Source: CAD feature listing. Evaluate the final solid. Frame: model axes, mm. A direction names the side the tool comes from. Round coordinates to 2 decimals unless told otherwise and drop trailing zeros. Write each loop counter-clockwise with the first axis right and the second up, starting at its lowest first coordinate (ties: lowest second). Pieces come first, ordered by that corner, then holes. Notation, with made-up numbers: M 86,37 L 129,37 A25 cw 129,72 Z; hole C -21,58.25 d10. An arc over 180 degrees is marked long. Use a Markdown table: item, result.
Autodesk Inventor part; units mm, degrees
ref_plane "YZ Plane" through (0, 0, 0) normal (1, 0, 0) x (0, 1, 0)
ref_plane "XZ Plane" through (0, 0, 0) normal (0, 1, 0) x (-1, 0, 0)
ref_plane "XY Plane" through (0, 0, 0) normal (0, 0, 1) x (1, 0, 0)
sketch "Sketch1" plane through (0, 0, 0) normal (0, 0, 1) x (1, 0, 0)
  line L0 (0, 0) -> (0, 12.75) construction
  line L1 (0, 0) -> (13.9342, 0) construction
  line L2 (0, 0) -> (0, -3)
  line L3 (0, -3) -> (12.5, -3)
  line L4 (12.5, -3) -> (12.5, 3.25)
  line L5 (12.5, 3.25) -> (9.075, 3.25)
  line L6 (9.075, 3.25) -> (9.075, 0)
  line L7 (9.075, 0) -> (0, 0)
  line L8 (3, 0) -> (5, 0)
  line L9 (5, 0) -> (5, -0.5)
  line L10 (5, -0.5) -> (3, -0.5)
  line L11 (3, -0.5) -> (3, 0)
  dimension "d0" = 3
  dimension "d1" = 5
  dimension "d2" = 0.5
  dimension "d3" = 9.075
  dimension "d4" = 12.5
  dimension "d5" = 3.25
  dimension "d6" = 3
revolve "Revolution1" add sketch "Sketch1" angle 360 about axis through (0, 0, 0) along (0, 1, 0) contours L7 L11 L10 L9 L6 L5 L4 L3 L2
chamfer "Chamfer1" distance 2 angle 45 1 edges at (-12.5, -3, 0)
chamfer "Chamfer2" distance 1 angle 45 1 edges at (-12.5, 3.25, 0)
sketch "Sketch2" plane through (0, 3.25, 0) normal (0, 1, 0) x (1, 0, 0)
  circle A0 centre (0, 0) radius 12.5
  circle A1 centre (0, 0) radius 12.5
  circle A2 centre (0, -12.5) radius 2.5
  line L0 (0, 0) -> (0, -12.5) construction
  point P0 (2.4875, -12.25)
  point P1 (-2.4875, -12.25)
  dimension "d14" = 5
extrude "Extrusion1" cut sketch "Sketch2" against normal through all contours A2 A0 picked at (0, -11.6481)
pattern_circular "Circular Pattern1" count 4 over 360 about axis through (0, -10, 0) along (0, 1, 0) of "Extrusion1"
sketch "Sketch3" plane through (0, 3.25, 12.5) normal (0, 1, 0) x (1, 0, 0)
  line L0 (0, 12.5) -> (0, -7.7808) construction
  line L1 (0, 12.5) -> (13.1543, -0.6543) construction
  circle A0 centre (7.4246, 5.0754) radius 0.75
  dimension "d20" = 45
  dimension "d21" = 1.5
  dimension "d22" = 10.5
extrude "Extrusion2" add sketch "Sketch3" along normal blind 1.5
chamfer "Chamfer3" distance 0.35 angle 45 1 edges at (6.6746, 4.75, 7.4246)
pattern_circular "Circular Pattern2" count 4 over 360 about axis through (0, -10, 0) along (0, 1, 0) of "Extrusion2", "Chamfer3"
properties part number "cpd_1.9_p0_v12"
Q1. Line query: L1, parallel to X at y = -0.15, z = 0; L2, parallel to Z at x = 0, y = 2.25 (3 decimals). Output: solid intervals per line, ascending.
Results are:
| item | result |
|---|---|
| L1 | -10 to -5, -3 to 3, 5 to 10 |
| L2 | -10 to -9.075, 9.075 to 10 |
Q2. Mould query, pull axis Z, two halves, no side actions, for faces 1 (the flat face through (0, -3, 0)), 2 (the conical face through (8.186, 3.076, -8.323)), 3 (the cylindrical face through (0, 0, 10)), 4 (the cylindrical face through (-1.08, -0.25, -4.88)). Classes: +Z half, -Z half, draft (parallel to the pull), parting line (faces both ways), or undercut.
Results are:
| item | result |
|---|---|
| face 1 | draft |
| face 2 | -Z half |
| face 3 | +Z half |
| face 4 | undercut |
Q3. Section C-C on z = 0. Return loops of the section in (x, y) (3 decimals).
Results are:
| item | result |
|---|---|
| outline | M -10,-3 L 10,-3 L 10,3.25 L 9.075,3.25 L 9.075,0 L 5,0 L 5,-0.5 L 3,-0.5 L 3,0 L -3,0 L -3,-0.5 L -5,-0.5 L -5,0 L -9.075,0 L -9.075,3.25 L -10,3.25 Z |
Q4. Section A-A on x = 0. Return loops of the section in (y, z) (3 decimals).
Results are:
| item | result |
|---|---|
| outline | M -3,-10 L 3.25,-10 L 3.25,-9.075 L 0,-9.075 L 0,-5 L -0.5,-5 L -0.5,-3 L 0,-3 L 0,3 L -0.5,3 L -0.5,5 L 0,5 L 0,9.075 L 3.25,9.075 L 3.25,10 L -3,10 Z |
Q5. First-contact query: pin 1 Ø11.5 at (x, z) = (0, 0) entering from +Y; pin 2 Ø3 at (x, y) = (7, 2.5) entering from +Z; pin 3 Ø2 at (x, y) = (8, 1.5) entering from -Z. Flat tips, straight axial feed; report the tip coordinate or a pass-through.
Results are:
| item | result |
|---|---|
| pin 1 | y = 0 |
| pin 2 | z = 11.21 |
| pin 3 | z = -10.36 |
Q6. Reachability of faces 5 (the flat face through (4, 0, 4)), 6 (the conical face through (-7.9, -2.4, 7.8)) from +Z, -Z, +X, -X, +Y, -Y: full face, straight path, thin tool, end or side. Return the list, or none.
Results are:
| item | result |
|---|---|
| face 5 | +Y |
| face 6 | +Z, -X, -Y |
Q7. Section B-B on y = 1.75. Return loops of the section in (x, z) (3 decimals).
Results are:
| item | result |
|---|---|
| outline | M -12.25,-2.487 A12.5 ccw -2.487,-12.25 A2.5 cw 2.487,-12.25 A12.5 ccw 12.25,-2.487 A2.5 cw 12.25,2.487 A12.5 ccw 2.487,12.25 A2.5 cw -2.487,12.25 A12.5 ccw -12.25,2.487 A2.5 cw Z; hole C 0,0 d18.15 |
